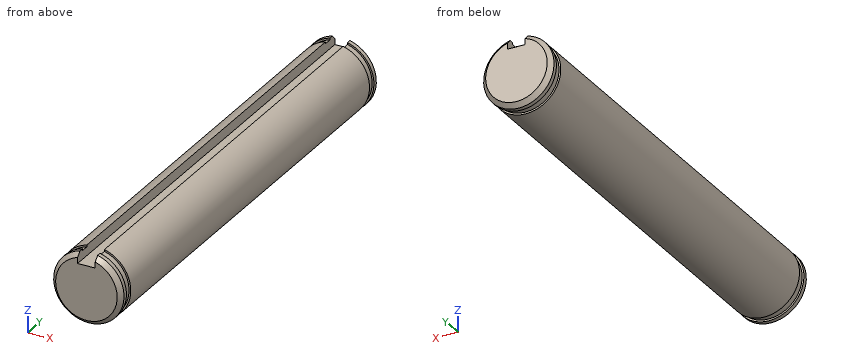
```python
from build123d import *

# Parameters (mm, degrees)
F0_R      = 4
F1_DEPTH  = 53
F2_W      = 2
F2_H      = 2.6729833462
F3_DEPTH  = 53.001
F4_SIZE   = 0.5
F6_R      = 5.1282432724
F6_R_2    = 3.8
F7_DEPTH  = 0.9
F9_R      = 7.9440327168
F9_R_2    = 3.8
F10_DEPTH = 0.9


with BuildPart() as f1:
    # F0 (on Front) → F1 (new body)
    with BuildSketch(Plane.XZ):
        Circle(F0_R)
    extrude(amount=F1_DEPTH)

    # F2 (on face) → F3 (cut, through all)
    with BuildSketch(Plane.XZ.offset(53)):
        with Locations((0, 4.0094750193)):
            Rectangle(F2_W, F2_H)
    extrude(amount=-F3_DEPTH, mode=Mode.SUBTRACT)

    # F4
    f4_edges = [f1.edges().sort_by_distance(p)[0] for p in [
        (0, -53, -4),
        (0, 0, -4),
    ]]
    chamfer(f4_edges, length=F4_SIZE)

    # F6 (on offset) → F7 (cut)
    with BuildSketch(Plane.XZ.offset(52)):
        Circle(F6_R)
        Circle(F6_R_2, mode=Mode.SUBTRACT)
    extrude(amount=-F7_DEPTH, mode=Mode.SUBTRACT)

    # F9 (on offset) → F10 (cut)
    with BuildSketch(Plane(origin=(0, -1, 0), x_dir=(-1, 0, 0), z_dir=(0, 1, 0))):
        Circle(F9_R)
        Circle(F9_R_2, mode=Mode.SUBTRACT)
    extrude(amount=-F10_DEPTH, mode=Mode.SUBTRACT)


solid = f1.part
```
CAD build for the part. Positions are in the model's coordinates, mm. Round coordinates to 2 decimals unless told otherwise and drop trailing zeros. Order: outer loops, then holes, each group sorted by start corner. A loop starts at its lowest first (then second) coordinate and runs counter-clockwise, first axis right, second up. Notation, with made-up numbers: (80, -39) - (100, -39) arc R20 cw to (100, -12) - close; hole circle Ø2 at (-10, -35). An arc over 180 degrees is marked (long way). Answer in a Markdown table with one row per item. Add a question column.
(1) Drop flat-ended pins along their axis: pin 1 Ø3 at (y, z) = (-20.5, 3) entering from -X; pin 2 Ø0.6 at (x, y) = (0, -28.5) entering from +Z; pin 3 Ø1 at (x, z) = (0, 1.5) entering from +Y; pin 4 Ø1.3 at (y, z) = (-14.5, 3.5) entering from +X. Give the stop position or say it passes through.
(2) Band-saw the part on A-A on x = 0. List the corners of the cut face in (y, z).
(3) Band-saw the part on B-B on y = -20.5. List the corners of the cut face in (x, z).
(4) Probe L1, parallel to Y at x = -3, z = 2.5; L2, parallel to Z at x = 1.25, y = -46.5; L3, parallel to X at y = -49, z = 3. List the from-to ranges inside material, lowest first. Write a range as [from, to].
Data:
| question | item | result |
|---|---|---|
| 1 | pin 1 | stops at x = -3.71 |
| 1 | pin 2 | stops at z = 2.67 |
| 1 | pin 3 | stops at y = 0 |
| 1 | pin 4 | stops at x = 2.81 |
| 2 | outline | (-53, -3.5) - (-52.5, -4) - (-52, -4) - (-52, -3.8) - (-51.1, -3.8) - (-51.1, -4) - (-1.9, -4) - (-1.9, -3.8) - (-1, -3.8) - (-1, -4) - (-0.5, -4) - (0, -3.5) - (0, 2.67) - (-53, 2.67) - close |
| 3 | outline | (-1, 2.67) - (-1, 3.87) arc R4 ccw (long way) to (1, 3.87) - (1, 2.67) - close |
| 4 | L1 | y = [-52.59, -52], [-51.1, -1.9], [-1, -0.41] |
| 4 | L2 | z = [-3.8, 3.8] |
| 4 | L3 | x = [-2.65, -1], [1, 2.65] |
